```python
from build123d import *

# Parameters (mm, degrees)
BOSS_EXTRUDE1_DEPTH   = 16
BOSS_EXTRUDE1_2_DEPTH = 16
SKETCH2_W             = 32.4
SKETCH2_H             = 6.7
BOSS_EXTRUDE2_DEPTH   = 2
CHAMFER1_SIZE         = 0.5
CHAMFER1_SIZE2        = 4.072173214
CHAMFER1_PART_2_SIZE  = 0.5
CHAMFER1_PART_2_SIZE2 = 4.072173214
CHAMFER4_SIZE         = 0.5
SKETCH4_RX            = 0.75
SKETCH4_RY            = 0.1
BOSS_EXTRUDE3_DEPTH   = 2
SKETCH5_RX            = 0.75
SKETCH5_RY            = 0.1
BOSS_EXTRUDE4_DEPTH   = 2


with BuildPart() as part:
    # Sketch1 → Boss-Extrude1 (new body)
    with BuildSketch(Plane(origin=(0, 0, 0), x_dir=(1, 0, 0), z_dir=(0, 1, 0))):
        Polygon((-14.2, 0.85), (-16.2, 0.85), (-16.2, 3.35), (16.2, 3.35), (16.2, 0.85), (14.2, 0.85), (14.2, 1.35), (-14.2, 1.35), align=None)
    extrude(amount=BOSS_EXTRUDE1_DEPTH)



with BuildPart() as body_2:
    # Sketch1 → Boss-Extrude1 2 (new body)
    with BuildSketch(Plane(origin=(0, 0, 0), x_dir=(1, 0, 0), z_dir=(0, 1, 0))):
        Polygon((-16.2, -3.35), (16.2, -3.35), (16.2, -0.85), (14.2, -0.85), (14.2, -1.35), (-14.2, -1.35), (-14.2, -0.85), (-16.2, -0.85), align=None)
    extrude(amount=BOSS_EXTRUDE1_2_DEPTH)


with BuildPart() as part_1:
    add(part.part)

    add(body_2.part)  # Boss-Extrude2 merges body 2
    # Sketch2 → Boss-Extrude2 (add)
    with BuildSketch(Plane(origin=(0, 16, 0), x_dir=(1, 0, 0), z_dir=(0, 1, 0))):
        Rectangle(SKETCH2_W, SKETCH2_H)
    extrude(amount=BOSS_EXTRUDE2_DEPTH)

    # Chamfer1
    chamfer1_edges = [part_1.edges().sort_by_distance(p)[0] for p in [
        (0, 0, 1.35),
    ]]
    chamfer1_side = [part_1.faces().sort_by_distance(p)[0] for p in [
        (0, 0, 2.31257485),
    ]]
    chamfer(chamfer1_edges, length=CHAMFER1_SIZE, length2=CHAMFER1_SIZE2, reference=chamfer1_side[0])

    # Chamfer1 part 2
    chamfer1_part_2_edges = [part_1.edges().sort_by_distance(p)[0] for p in [
        (0, 0, -1.35),
    ]]
    chamfer1_part_2_side = [part_1.faces().sort_by_distance(p)[0] for p in [
        (0, 0, -2.31257485),
    ]]
    chamfer(chamfer1_part_2_edges, length=CHAMFER1_PART_2_SIZE, length2=CHAMFER1_PART_2_SIZE2, reference=chamfer1_part_2_side[0])

    # Chamfer4
    chamfer4_edges = [part_1.edges().sort_by_distance(p)[0] for p in [
        (0, 0, -3.35),
        (0, 0, 3.35),
    ]]
    chamfer(chamfer4_edges, length=CHAMFER4_SIZE)

    # Sketch4 → Boss-Extrude3 (add)
    with BuildSketch(Plane(origin=(16.2, 0, 0), x_dir=(0, 0, -1), z_dir=(1, 0, 0))):
        with Locations(Location((-0.85, 0.75), (0, 0, 90))):
            Ellipse(SKETCH4_RX, SKETCH4_RY)
        with Locations(Location((0.85, 0.75), (0, 0, 90))):
            Ellipse(SKETCH4_RX, SKETCH4_RY)
    extrude(amount=-BOSS_EXTRUDE3_DEPTH)

    # Sketch5 → Boss-Extrude4 (add)
    with BuildSketch(Plane.ZY.offset(16.2)):
        with Locations(Location((-0.85, 0.75), (0, 0, -90))):
            Ellipse(SKETCH5_RX, SKETCH5_RY)
        with Locations(Location((0.85, 0.75), (0, 0, -90))):
            Ellipse(SKETCH5_RX, SKETCH5_RY)
    extrude(amount=-BOSS_EXTRUDE4_DEPTH)


solid = part_1.part
```
Could you check a few things on this model? Use its own coordinates, in mm. A direction names the side the tool comes from. Coordinates: 2 decimals unless noted, no trailing zeros. Order: outer loops, then holes, each group sorted by start corner. A loop starts at its lowest first (then second) coordinate and runs counter-clockwise, first axis right, second up. Notation, with made-up numbers: M -36.5,15 L 11.5,15 A12 ccw 11.5,33 Z; hole C -1.5,75 d7. An arc over 180 degrees is marked long. Use a Markdown table: item, result. Add a question column.
Q1. I want a section at A-A on y = 15. List the corners of the cut face in (x, z) for me.
Q2. We'd pull the mould along X, two halves only. Please class faces 4 (the flat face through (0, 10, 1.35)), 5 (the flat face through (15, 9, 0.85)), 6 (the flat face through (-16.2, 9, 2)): pulls with the +X half, pulls with the -X half, needs draft (parallel to the pull), parting line crosses it, or undercut.
Q3. If I drill on L1, parallel to Z at x = 1.5, y = 5.5; L2, parallel to X at y = 15, z = 1; L3, parallel to Y at x = 1.5, z = -1.25, over which ranges is the centre line in solid material (lowest first)?
Q4. I'm going to push a flat-ended pin straight in: pin 1 (1.4 mm diameter, centred on x = 4, z = 0.5, fed in from -Y). Where does the tip first touch, or does it pass through?
Q5. Which directions (+Z, -Z, +X, -X, +Y, -Y) give clear straight access to the entire face, cutting with the end or side of a thin tool? Please do faces 1 (the flat face through (-15, 9, 0.85)), 2 (the flat face through (0.199, 2.065, 1.597)), 3 (the flat face through (-0.2, 0, 2.3)).
Q6. I want a section at D-D on y = 3.5. List the corners of the cut face in (x, z) for me, then the cut area to 3 significant figures.
Q7. I want a section at B-B on x = 1.5. List the corners of the cut face in (y, z) for me, then the cut area to 3 significant figures.
Q8. I want a section at C-C on z = 0. List the corners of the cut face in (x, y) for me, then the cut area to 3 significant figures.
Checked values:
| question | item | result |
|---|---|---|
| 1 | outline | M -16.2,-3.35 L 16.2,-3.35 L 16.2,-0.85 L 14.2,-0.85 L 14.2,-1.35 L -14.2,-1.35 L -14.2,-0.85 L -16.2,-0.85 Z; M -16.2,0.85 L -14.2,0.85 L -14.2,1.35 L 14.2,1.35 L 14.2,0.85 L 16.2,0.85 L 16.2,3.35 L -16.2,3.35 Z |
| 2 | face 4 | undercut |
| 2 | face 5 | needs draft |
| 2 | face 6 | pulls with the -X half |
| 3 | L1 | -3.35 to -1.35, 1.35 to 3.35 |
| 3 | L2 | -16.2 to -14.2, 14.2 to 16.2 |
| 3 | L3 | 16 to 18 |
| 4 | pin 1 | y = 16 |
| 5 | face 1 | +X, -X |
| 5 | face 2 | -Y |
| 5 | face 3 | +Z, -Z, +X, -X, -Y |
| 6 | outline | M -16.2,-3.35 L 16.2,-3.35 L 16.2,-0.85 L 14.2,-0.85 L 14.2,-1.42 L -14.2,-1.42 L -14.2,-0.85 L -16.2,-0.85 Z; M -16.2,0.85 L -14.2,0.85 L -14.2,1.42 L 14.2,1.42 L 14.2,0.85 L 16.2,0.85 L 16.2,3.35 L -16.2,3.35 Z |
| 6 | area | 130 mm² |
| 7 | outline | M 0,-2.85 L 0.5,-3.35 L 18,-3.35 L 18,3.35 L 0.5,3.35 L 0,2.85 L 0,1.85 L 4.07,1.35 L 16,1.35 L 16,-1.35 L 4.07,-1.35 L 0,-1.85 Z |
| 7 | area | 75.1 mm² |
| 8 | outline | M -16.2,16 L 16.2,16 L 16.2,18 L -16.2,18 Z |
| 8 | area | 64.8 mm² |
